The listing builds one solid part. Answer for the finished solid, in the listing's coordinates (mm). A direction names the side the tool comes from. Give positions to 0.01 mm unless a question says otherwise; leave off trailing zeros. Write each loop counter-clockwise with the first axis right and the second up, starting at its lowest first coordinate (ties: lowest second). Pieces come first, ordered by that corner, then holes. Notation, with made-up numbers: (22.25, 7) -> (67.25, 7) arc R30 ccw to (67.25, 37) -> close; hole circle Ø4 at (22, 4). An arc over 180 degrees is marked (long way). Put each result on its own line as item: value. Start each with the question number.
1) A cutting plane is placed at C-C (y = -0.9). Write down the section's boundary in (x, z), then the cut area to 3 significant figures.
2) A cutting plane is placed at B-B (z = -3.5). Write down the section's boundary in (x, y), then the cut area to 3 significant figures.
3) For faces 1 (the flat face through (20.96, -0.99, -37.28)), 2 (the flat face through (-1, 0, 45)), determine the directions among +Z, -Z, +X, -X, +Y, -Y from which every point of the face is accessible in a straight line to the end or side of a thin tool.
4) A cutting plane is placed at A-A (x = -48). Write down the section's boundary in (y, z), then the cut area to 3 significant figures.
5) Find the intervals of material crossed by line 1 along Z through (x, y) = (-37.5, -0.55); line 2 along Z through (x, y) = (-53, -0.1); line 3 along X through (y, z) = (-1.6, -10), in increasing order. Write a range as from..to.
6) For a pull along X with two mould halves and no side action, classify faces 3 (the flat face through (-20.96, -0.99, 37.28)), 4 (the flat face through (-1, -2, 45)) as released by +X, released by -X, zero draft, split by the parting line, or undercut.
from build123d import *

# Parameters (mm, degrees)
F0_W     = 130
F0_H     = 100
F0_R     = 0.5
F1_DEPTH = 2


with BuildPart() as f1:
    # F0 (on Front) → F1 (new body)
    with BuildSketch(Plane.XZ):
        Rectangle(F0_W, F0_H)
        with Locations((-37.5, -37.5)):
            Circle(F0_R, mode=Mode.SUBTRACT)
        with Locations((37.5, -37.5)):
            Circle(F0_R, mode=Mode.SUBTRACT)
        with Locations((-37.5, 37.5)):
            Circle(F0_R, mode=Mode.SUBTRACT)
        Polygon((-27.489878, 30.75), (-14.239878, 44), (0, 44), (14.239878, 44), (27.489878, 30.75), (56.5, 30.75), (56.5, 0), (56.5, -30.75), (27.489878, -30.75), (14.239878, -44), (0, -44), (-14.239878, -44), (-27.489878, -30.75), (-56.5, -30.75), (-56.5, 0), (-56.5, 30.75), align=None, mode=Mode.SUBTRACT)
        with Locations((37.5, 37.5)):
            Circle(F0_R, mode=Mode.SUBTRACT)
    extrude(amount=F1_DEPTH)


solid = f1.part
Reply:
1. outline: (-65, -50) -> (65, -50) -> (65, 50) -> (-65, 50) -> close; hole (-56.5, -30.75) -> (-27.49, -30.75) -> (-14.24, -44) -> (14.24, -44) -> (27.49, -30.75) -> (56.5, -30.75) -> (56.5, 30.75) -> (27.49, 30.75) -> (14.24, 44) -> (-14.24, 44) -> (-27.49, 30.75) -> (-56.5, 30.75) -> close; hole circle Ø1 at (-37.5, -37.5); hole circle Ø1 at (-37.5, 37.5); hole circle Ø1 at (37.5, -37.5); hole circle Ø1 at (37.5, 37.5)
1. area: 4,940 mm2
2. outline: (-65, -2) -> (-56.5, -2) -> (-56.5, 0) -> (-65, 0) -> close; (56.5, -2) -> (65, -2) -> (65, 0) -> (56.5, 0) -> close
2. area: 34.0 mm2
3. face 1: +Y, -Y
3. face 2: +Z, -Z, +X, -X, +Y
4. outline: (-2, -50) -> (0, -50) -> (0, -30.75) -> (-2, -30.75) -> close; (-2, 30.75) -> (0, 30.75) -> (0, 50) -> (-2, 50) -> close
4. area: 77.0 mm2
5. line 1: z = -50..-38, -37..-30.75, 30.75..37, 38..50
5. line 2: z = -50..-30.75, 30.75..50
5. line 3: x = -65..-56.5, 56.5..65
6. face 3: undercut
6. face 4: zero draft
